Work out the finished part from the listing and answer in its coordinate system (mm). Face numbers are marked on the shaded views. Give positions to 0.01 mm unless a question says otherwise; leave off trailing zeros. Loops run counter-clockwise (first coordinate to the right, second up) from the corner with the lowest first, then second, coordinate; pieces in that order, holes last. Notation, with made-up numbers: M 15,53.25 L 69,53.25 A22 cw 69,78.25 Z; hole C 9,-38.5 d10. An arc over 180 degrees is marked long. Write item = value, one per line. Start each with the question number.
1. The mould has two halves that part along Y. Classify the marked faces 1, 2, 3 and 4: released by +Y, released by -Y, zero draft, split by the parting line, or undercut.
2. A flat-ended cylindrical pin translates along its axis: pin 1 Ø6 at (y, z) = (6.35, -4.445) entering from +X. Find the tip coordinate at first contact, or state that the pin passes through.
3. Section C-C on z = 4.5 is taken. Give the number of separate pieces and of enclosed holes in the cut face, plus the area to 3 significant figures.
4. Section B-B on x = 3.5 is taken. Determine the outline of the cut face in (y, z) (3 decimals).
5. Section A-A on y = -12.7 is taken. Determine the outline of the cut face in (x, z) (3 decimals).
6. Consider L1, parallel to Y at x = 0.5, z = 4.5; L2, parallel to Y at x = 6, z = 2; L3, parallel to Z at x = 3.5, y = 8 (3 decimals). Determine where each line is inside the solid, lowest interval first. Write a range as [from, to].
```python
from build123d import *

# Parameters (mm, degrees)
SKETCH1_W           = 19.05
SKETCH1_H           = 38.1
SKETCH1_R           = 1.89865
BOSS_EXTRUDE1_DEPTH = 6.35
CHAMFER1_SIZE       = 2.00025
CHAMFER1_SIZE2      = 1.738790797


with BuildPart() as part:
    # Sketch1 → Boss-Extrude1 (new body)
    with BuildSketch(Plane(origin=(0, 0, 0), x_dir=(0, 0, -1), z_dir=(1, 0, 0))):
        Rectangle(SKETCH1_W, SKETCH1_H)
        with Locations((-4.445, 12.7)):
            Circle(SKETCH1_R, mode=Mode.SUBTRACT)
        with Locations((4.445, 6.35)):
            Circle(SKETCH1_R, mode=Mode.SUBTRACT)
        with Locations((-4.445, -12.7)):
            Circle(SKETCH1_R, mode=Mode.SUBTRACT)
        with Locations((4.445, -6.35)):
            Circle(SKETCH1_R, mode=Mode.SUBTRACT)
    extrude(amount=BOSS_EXTRUDE1_DEPTH)

    # Chamfer1
    chamfer1_edges = [part.edges().sort_by_distance(p)[0] for p in [
        (6.35, 12.7, 6.34365),
        (6.35, 6.35, -2.54635),
        (6.35, -12.7, 6.34365),
        (6.35, -6.35, -2.54635),
    ]]
    chamfer1_side = [part.faces().sort_by_distance(p)[0] for p in [
        (6.35, 0, 0),
    ]]
    chamfer(chamfer1_edges, length=CHAMFER1_SIZE, length2=CHAMFER1_SIZE2, reference=chamfer1_side[0])


solid = part.part
```
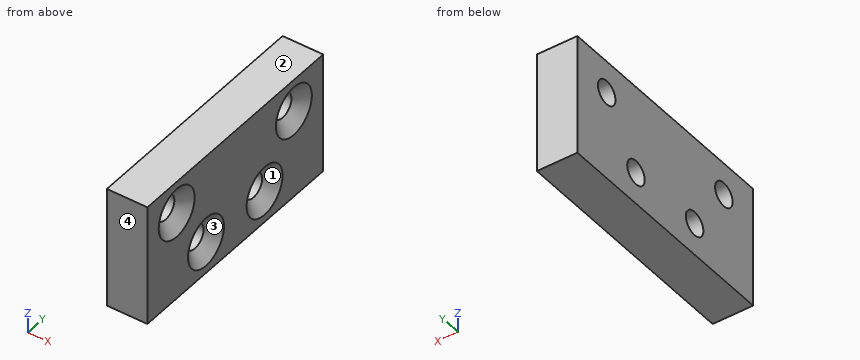
Verdict:
q1.face_1 = undercut
q1.face_2 = zero draft
q1.face_3 = undercut
q1.face_4 = released by -Y
q2.pin_1 = 5.57
q3.separate_pieces = 3
q3.enclosed_holes = 0
q3.area = 187 mm2
q4.outline = M -19.05,-9.525 L 19.05,-9.525 L 19.05,9.525 L -19.05,9.525 Z; hole C -12.7,4.445 d3.797; hole C -6.35,-4.445 d3.797; hole C 6.35,-4.445 d3.797; hole C 12.7,4.445 d3.797
q5.outline = M 0,-9.525 L 6.35,-9.525 L 6.35,0.546 L 4.611,2.546 L 0,2.546 Z; M 0,6.344 L 4.611,6.344 L 6.35,8.344 L 6.35,9.525 L 0,9.525 Z
q6.L1 = [-19.05, -14.6], [-10.8, 10.8], [14.6, 19.05]
q6.L2 = [-19.05, -15.2], [-10.2, 10.2], [15.2, 19.05]
q6.L3 = [-9.525, -5.384], [-3.506, 9.525]
